```python
from build123d import *

# Parameters (mm, degrees)
CROQUIS7_R              = 8
SALIENTE_EXTRUIR3_DEPTH = 5
CROQUIS4_R              = 9
SALIENTE_EXTRUIR4_DEPTH = 1
CROQUIS10_R             = 4
CORTAR_EXTRUIR2_DEPTH   = 5
REDONDEO1_R             = 0.25
REDONDEO2_R             = 0.1


with BuildPart() as part:
    # Croquis7 → Saliente-Extruir3 (new body)
    with BuildSketch(Plane(origin=(0, 0, 0), x_dir=(1, 0, 0), z_dir=(0, 1, 0))):
        with Locations(Location((0, 0, 0), (0, 0, 270))):
            Circle(CROQUIS7_R)
    extrude(amount=SALIENTE_EXTRUIR3_DEPTH)

    # Croquis4 → Saliente-Extruir4 (add)
    with BuildSketch(Plane(origin=(0, 0, 0), x_dir=(1, 0, 0), z_dir=(0, 1, 0))):
        with Locations(Location((0, 0, 0), (0, 0, 270))):
            Circle(CROQUIS4_R)
    extrude(amount=SALIENTE_EXTRUIR4_DEPTH)

    # Croquis10 → Cortar-Extruir2 (cut)
    with BuildSketch(Plane(origin=(0, 0, 0), x_dir=(1, 0, 0), z_dir=(0, 1, 0))):
        with Locations(Location((0, 0, 0), (0, 0, 270))):
            Circle(CROQUIS10_R)
    extrude(amount=CORTAR_EXTRUIR2_DEPTH, mode=Mode.SUBTRACT)

    # Redondeo1
    redondeo1_edges = [part.edges().sort_by_distance(p)[0] for p in [
        (0, 5, -4),
        (0, 5, -8),
    ]]
    fillet(redondeo1_edges, radius=REDONDEO1_R)

    # Redondeo2
    redondeo2_edges = [part.edges().sort_by_distance(p)[0] for p in [
        (0, 0, -9),
        (0, 1, -9),
    ]]
    fillet(redondeo2_edges, radius=REDONDEO2_R)


solid = part.part
```
Geometry check sheet. Reference: the model listing, model coordinates, mm. Coordinates: 2 decimals unless noted, no trailing zeros. Write each loop counter-clockwise with the first axis right and the second up, starting at its lowest first coordinate (ties: lowest second). Pieces come first, ordered by that corner, then holes. Notation, with made-up numbers: M 28.5,36.5 L 71.5,36.5 A23 cw 71.5,65.5 Z; hole C 88.25,8.5 d6. An arc over 180 degrees is marked long. Use one line per item in the form item = value. Start each with the question number.
1) Section check B-B on z = 0. Enter the section's corners in (x, y), and give its area (3 significant figures).
2) Section check A-A on x = 0. Enter the section's corners in (y, z), and give its area (3 significant figures).
3) Go/stop test with flat-tipped pins: pin 1 Ø1 at (y, z) = (3, -2.5) entering from +X; pin 2 Ø1 at (x, y) = (7, 3) entering from +Z; pin 3 Ø3 at (y, z) = (3, -2) entering from +X. Record where each tip stops, or that it passes through.
4) Release check for a two-part mould opening along X. For faces 1 (the cylindrical face through (-7.81, 2.85, -1.73)), 2 (the cylindrical face through (-3.905, 2.342, -0.867)), 3 (the flat face through (5, 1, -7)) record: pulls with the +X half, pulls with the -X half, needs draft (parallel to the pull), parting line crosses it, or undercut.
5) Section check C-C on y = 3.3. Enter the section's corners in (x, z), and give its area (3 significant figures).
6) Thickness scan on probe 1 along X at (y, z) = (2.9, 0); probe 2 along Z at (x, y) = (-1.25, 3.35); probe 3 along Y at (x, z) = (-3.25, -7.75). Record the ranges inside material, lowest first. Write a range as from..to.
Responses:
q1.outline = M -9,0.1 A0.1 ccw -8.9,0 L -4,0 L -4,4.75 A0.25 ccw -4.25,5 L -7.75,5 A0.25 ccw -8,4.75 L -8,1 L -8.9,1 A0.1 ccw -9,0.9 Z; M 4,0 L 8.9,0 A0.1 ccw 9,0.1 L 9,0.9 A0.1 ccw 8.9,1 L 8,1 L 8,4.75 A0.25 ccw 7.75,5 L 4.25,5 A0.25 ccw 4,4.75 Z
q1.area = 41.9 mm2
q2.outline = M 0,-8.9 A0.1 ccw 0.1,-9 L 0.9,-9 A0.1 ccw 1,-8.9 L 1,-8 L 4.75,-8 A0.25 ccw 5,-7.75 L 5,-4.25 A0.25 ccw 4.75,-4 L 0,-4 Z; M 0,4 L 4.75,4 A0.25 ccw 5,4.25 L 5,7.75 A0.25 ccw 4.75,8 L 1,8 L 1,8.9 A0.1 ccw 0.9,9 L 0.1,9 A0.1 ccw 0,8.9 Z
q2.area = 41.9 mm2
q3.pin_1 = 7.75
q3.pin_2 = 4.66
q3.pin_3 = 7.98
q4.face_1 = parting line crosses it
q4.face_2 = undercut
q4.face_3 = needs draft
q5.outline = C 0,0 d16; hole C 0,0 d8
q5.area = 151 mm2
q6.probe_1 = -8..-4, 4..8
q6.probe_2 = -7.9..-3.8, 3.8..7.9
q6.probe_3 = 0..1
